from build123d import *

# Parameters (mm, degrees)
SKETCH_3_R          = 2.5
CUT_EXTRUDE_1_DEPTH = 6
SKETCH_4_R          = 2.5
CUT_EXTRUDE_2_DEPTH = 6
CUT_EXTRUDE_START   = -6
SKETCH_5_R          = 2.5
CUT_EXTRUDE_3_DEPTH = 6
SKETCH_6_R          = 2.5
CUT_EXTRUDE_4_DEPTH = 6
SKETCH_7_R          = 2.5
CUT_EXTRUDE_5_DEPTH = 6
FILLET_1_R          = 0.5
FILLET_2_R          = 0.5
FILLET_3_R          = 0.5
FILLET_4_R          = 0.5


with BuildPart() as part:
    # 스케치2 → 회전1 (revolve)
    with BuildSketch(Plane.XY, mode=Mode.PRIVATE) as revolve_1_sk:
        Polygon((0, 0), (0, 20), (23, 20), (23, 10), (22, 10), (22, 8), (20, 8), (20, 4.5), (22, 4.5), (22, 0), align=None)
    revolve(revolve_1_sk.sketch.rotate(Axis((0, 0, 0), (0, 1, 0)), 90), axis=Axis((0, 0, 0), (0, 1, 0)))

    # 스케치3 → 컷-돌출1 (cut)
    with BuildSketch(Plane.ZY.offset(23)):
        with Locations((0, 15)):
            Circle(SKETCH_3_R)
    extrude(amount=-CUT_EXTRUDE_1_DEPTH, mode=Mode.SUBTRACT)

    # 스케치4 → 컷-돌출2 (cut)
    with BuildSketch(Plane(origin=(0, 0, -23), x_dir=(-1, 0, 0), z_dir=(0, 0, -1))):
        with Locations((0, 15)):
            Circle(SKETCH_4_R)
    extrude(amount=-CUT_EXTRUDE_2_DEPTH, mode=Mode.SUBTRACT)

    # 스케치5 → 컷-돌출3 (cut)
    with BuildSketch(Plane(origin=(23, 0, 0), x_dir=(0, 0, -1), z_dir=(1, 0, 0)).offset(CUT_EXTRUDE_START)):
        with Locations(Location((0, 15, 0), (0, 0, 180))):
            Circle(SKETCH_5_R)
    extrude(amount=CUT_EXTRUDE_3_DEPTH, mode=Mode.SUBTRACT)

    # 스케치6 → 컷-돌출4 (cut)
    with BuildSketch(Plane.XY.offset(23).offset(CUT_EXTRUDE_START)):
        with Locations(Location((0, 15, 0), (0, 0, 180))):
            Circle(SKETCH_6_R)
    extrude(amount=CUT_EXTRUDE_4_DEPTH, mode=Mode.SUBTRACT)

    # 스케치7 → 컷-돌출5 (cut)
    with BuildSketch(Plane(origin=(0, 20, 0), x_dir=(1, 0, 0), z_dir=(0, 1, 0))):
        with Locations(Location((0, 0, 0), (0, 0, 270))):
            Circle(SKETCH_7_R)
    extrude(amount=-CUT_EXTRUDE_5_DEPTH, mode=Mode.SUBTRACT)

    # 필렛1
    fillet_1_edges = [part.edges().sort_by_distance(p)[0] for p in [
        (0, 8, 22),
    ]]
    fillet(fillet_1_edges, radius=FILLET_1_R)

    # 필렛2
    fillet_2_edges = [part.edges().sort_by_distance(p)[0] for p in [
        (0, 4.5, 22),
    ]]
    fillet(fillet_2_edges, radius=FILLET_2_R)

    # 필렛3
    fillet_3_edges = [part.edges().sort_by_distance(p)[0] for p in [
        (0, 0, 22),
    ]]
    fillet(fillet_3_edges, radius=FILLET_3_R)

    # 필렛4
    fillet_4_edges = [part.edges().sort_by_distance(p)[0] for p in [
        (0, 10, 23),
    ]]
    fillet(fillet_4_edges, radius=FILLET_4_R)


solid = part.part
Input: part model. Units: mm. Frame: model coordinates. A direction names the side the tool comes from. Coordinates: 2 decimals unless noted, no trailing zeros. Order: outer loops, then holes, each group sorted by start corner. A loop starts at its lowest first (then second) coordinate and runs counter-clockwise, first axis right, second up. Notation, with made-up numbers: M -31,77 L 3,77 A4 ccw 3,83 Z; hole C -33.5,61.25 d9. An arc over 180 degrees is marked long. Answer as CSV lines item,"result".
1. Section A-A (y = 15). Return the cut outline in (x, z), then the cut area to 3 significant figures.
Reported:
outline,"M -22.86,-2.5 A23 ccw -2.5,-22.86 L -2.5,-17 L 2.5,-17 L 2.5,-22.86 A23 ccw 22.86,-2.5 L 17,-2.5 L 17,2.5 L 22.86,2.5 A23 ccw 2.5,22.86 L 2.5,17 L -2.5,17 L -2.5,22.86 A23 ccw -22.86,2.5 L -17,2.5 L -17,-2.5 Z; hole C 0,0 d5"
area,"1,520 mm2"
2. Material intervals for line 1 (Y direction, x = 21, z = 0); line 2 (Y direction, x = 10.5, z = -18); line 3 (X direction, y = 18.4, z = 0), sorted ascending. Write a range as from..to.
Reported:
line 1,"0..4.5, 8..12.5, 17.5..20"
line 2,"0..4.5, 8..20"
line 3,"-23..-2.5, 2.5..23"
3. Section B-B (y = 2.5). Return the cut outline in (x, z), then the cut area to 3 significant figures.
Reported:
outline,"C 0,0 d44"
area,"1,520 mm2"
4. First-contact query: P1, Ø2.5, axis at y = 15, z = -0.5, coming from the -X side; P2, Ø3, axis at y = 9, z = -5, coming from the -X side; P3, Ø1.5, axis at x = 0.5, y = 16, coming from the -Z side. Flat tips, straight axial feed; report the tip coordinate or a pass-through.
Reported:
P1,"x = -17"
P2,"x = -22.56"
P3,"z = -17"
5. Pull-direction query (Y, two-part tool) for faces 1 (the cylindrical face through (21.477, 2.226, 4.769)), 2 (the flat face through (19.9, 10, -9.9)), 3 (the cylindrical face through (-0.88, 6.23, 19.98)); classes: released by +Y, released by -Y, zero draft, split by the parting line, or undercut.
Reported:
face 1,"zero draft"
face 2,"released by -Y"
face 3,"undercut"
6. Access query for faces 4 (the flat face through (13, 4.5, 16)), 5 (the flat face through (17, 15, 0)), 6 (the cylindrical face through (-20.04, 12.56, -0.54)). Directions: +Z, -Z, +X, -X, +Y, -Y. A direction counts if a zero-diameter tool reaches every point of the face in a straight line with its end or side. Return the directions, or none.
Reported:
face 4,"none"
face 5,"+X"
face 6,"-X"
7. Section C-C (y = 18.25). Return the cut outline in (x, z), then the cut area to 3 significant figures.
Reported:
outline,"C 0,0 d46; hole C 0,0 d5"
area,"1,640 mm2"
